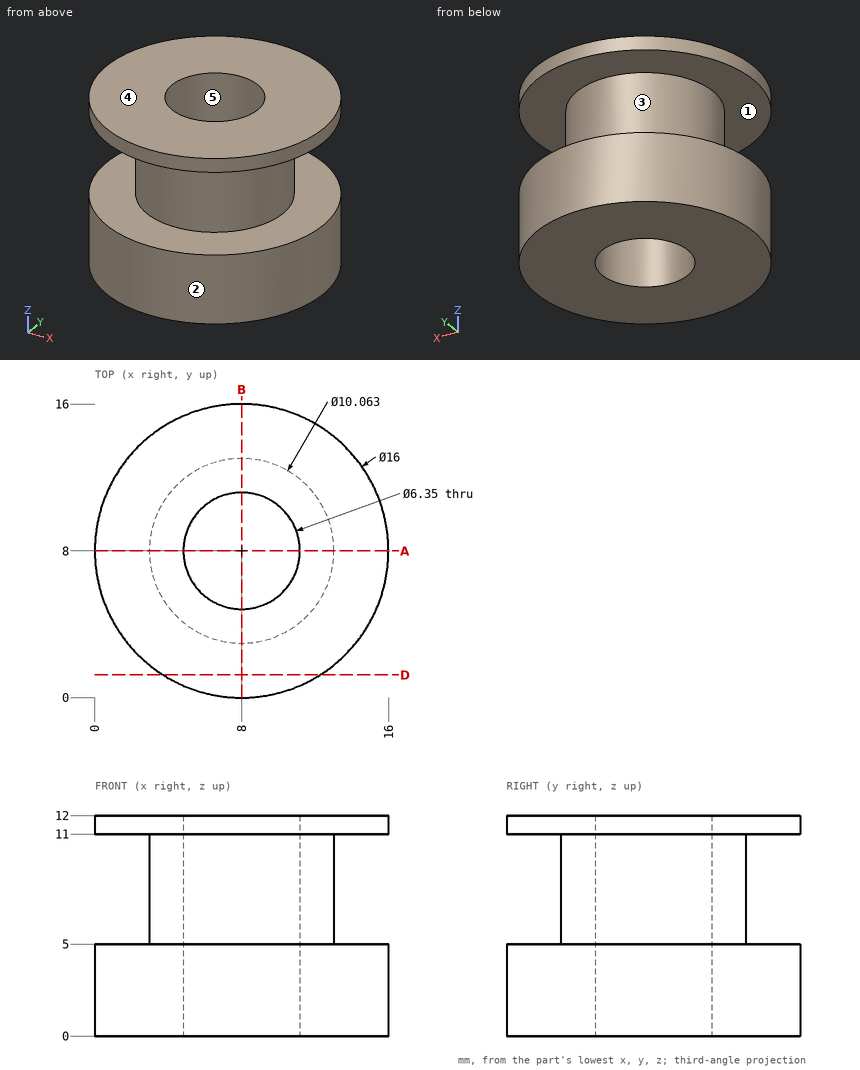
For this review, use the dimensioned drawing (mm, ordinates from the lowest corner) and the shaded views. A direction names the side the tool comes from. Round coordinates to 2 decimals unless told otherwise and drop trailing zeros. Write each loop counter-clockwise with the first axis right and the second up, starting at its lowest first coordinate (ties: lowest second). Pieces come first, ordered by that corner, then holes. Notation, with made-up numbers: (35.5, 19.25) - (79.5, 19.25) arc R21 cw to (79.5, 26.25) - close; hole circle Ø8 at (9, 72). An arc over 180 degrees is marked (long way). One line per item, written item: value. Start each with the question number.
1. Consider section A-A on y = 8. Write out the cut boundary in (x, z) (1 decimal).
2. Clearance check with flat-ended pins moving along their axes: P1, Ø2, axis at y = 6, z = 8, coming from the +X side; P2, Ø5, axis at x = 11, z = 10.5, coming from the -Y side. State where each tip first meets the part, or that it passes through.
3. To check wall thickness, follow L1, parallel to Y at x = 8, z = 6.75 (1 decimal); L2, parallel to Y at x = 8, z = 3.25 (1 decimal); L3, parallel to Z at x = 2.25, y = 12.25. State the ranges of each line that lie inside material, in increasing order. Write a range as from..to.
4. The part is to be moulded in two halves that separate along Y. For the marked faces 3, 4 and 5, say which applies: released by +Y, released by -Y, zero draft, split by the parting line, or undercut.
5. Machinability: for the marked faces 1 and 2, which of the approach directions +Z, -Z, +X, -X, +Y, -Y give a long, thin tool a straight path to every point of the face, cutting with its end or side? Answer none if there is none.
6. Consider section D-D on y = 1.25. Write out the cut boundary in (x, z).
Checks:
1. outline: (0, 0) - (4.8, 0) - (4.8, 12) - (0, 12) - (0, 11) - (3, 11) - (3, 5) - (0, 5) - close; (11.2, 0) - (16, 0) - (16, 5) - (13, 5) - (13, 11) - (16, 11) - (16, 12) - (11.2, 12) - close
2. P1: stops at x = 12.93
2. P2: stops at y = 0.02
3. L1: y = 3..4.8, 11.2..13
3. L2: y = 0..4.8, 11.2..16
3. L3: z = 0..5, 11..12
4. face 3: split by the parting line
4. face 4: zero draft
4. face 5: undercut
5. face 1: none
5. face 2: +Z, -Z
6. outline: (3.71, 0) - (12.29, 0) - (12.29, 5) - (3.71, 5) - close; (3.71, 11) - (12.29, 11) - (12.29, 12) - (3.71, 12) - close
